Here's the drawing with two shaded views (mm, measured from the low corner). I have some questions. A direction names the side the tool comes from. Coordinates: 2 decimals unless noted, no trailing zeros. Write each loop counter-clockwise with the first axis right and the second up, starting at its lowest first coordinate (ties: lowest second). Pieces come first, ordered by that corner, then holes.
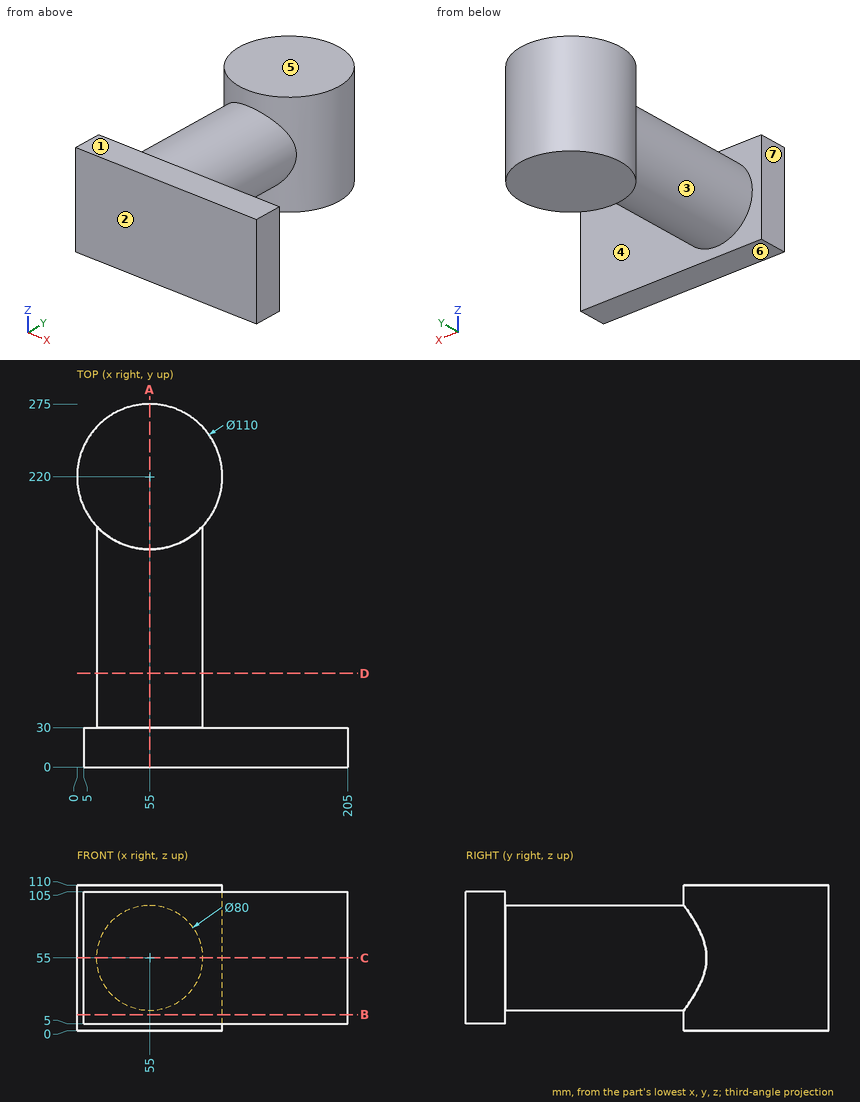
1. I want a section at C-C on z = 55. Please give me the cut outline in (x, y), plus the area to 3 significant figures.
Verdict:
outline: (5, 0) - (205, 0) - (205, 30) - (95, 30) - (95, 182.25) arc R55 ccw (long way) to (15, 182.25) - (15, 30) - (5, 30) - close
area: 26,700 mm2
2. Please list where these lines run through material, in increasing order: line 1 along Y through (x, z) = (54, 62); line 2 along Y through (x, z) = (52.5, 97); line 3 along Y through (x, z) = (173, 73.5).
Verdict:
line 1: y = 0 to 274.99
line 2: y = 0 to 30, 165.06 to 274.94
line 3: y = 0 to 30
3. I want a section at B-B on z = 12. Please give me the cut outline in (x, y).
Verdict:
outline: circle Ø110 at (55, 220); (5, 0) - (205, 0) - (205, 30) - (5, 30) - close
4. I want a section at D-D on y = 71. Please give me the cut outline in (x, z).
Verdict:
outline: circle Ø80 at (55, 55)
5. I want a section at A-A on x = 55. Please give me the cut outline in (y, z).
Verdict:
outline: (0, 5) - (30, 5) - (30, 15) - (165, 15) - (165, 0) - (275, 0) - (275, 110) - (165, 110) - (165, 95) - (30, 95) - (30, 105) - (0, 105) - close
6. If we mould it in two halves opening along Y, with no side actions, what happens to the marked faces 1, 2, 3 and 4? For each: pulls with the +Y half, pulls with the -Y half, needs draft (parallel to the pull), parting line crosses it, or undercut.
Verdict:
face 1: needs draft
face 2: pulls with the -Y half
face 3: undercut
face 4: undercut
7. On a 3-axis mill with a long thin cutter (end or side, diameter ignored), from which of +Z, -Z, +X, -X, +Y, -Y can I reach the whole of each face in a straight line? I mean the marked faces 5, 6 and 7. Say none if no direction works.
Verdict:
face 5: +Z, +X, -X, +Y, -Y
face 6: -Z, +X, -X, -Y
face 7: +Z, -Z, -X, -Y
8. For pin 1 (15 mm diameter, centred on y = 20, z = 45, fed in from -X); pin 2 (8 mm diameter, centred on x = 38.5, z = 68, fed in from +Y); pin 3 (12 mm diameter, centred on y = 59, z = 28.5, fed in from +X), each with a flat end and sliding along its axis, tell me the tip position at first contact or that it passes through.
Verdict:
pin 1: stops at x = 5
pin 2: stops at y = 273.56
pin 3: stops at x = 89.35
